For this review, take the finished solid that the model builds, in its own axes (mm). A direction names the side the tool comes from. Give positions to 0.01 mm unless a question says otherwise; leave off trailing zeros. Loops run counter-clockwise (first coordinate to the right, second up) from the corner with the lowest first, then second, coordinate; pieces in that order, holes last. Notation, with made-up numbers: (42.5, -7) - (80.5, -7) arc R23 cw to (80.5, 6) - close; hole circle Ø4 at (33.5, 14). An arc over 180 degrees is marked (long way). Put each result on its own line as item: value. Start each with the question number.
from build123d import *

# Parameters (mm, degrees)
CYLINDER_R              = 3.8
CYLINDER_DEPTH          = 50
CYLINDER001_R           = 10
CYLINDER001_DEPTH       = 15
BOX001_W                = 12
BOX001_H                = 12
BOX001_DEPTH            = 10
BODY003_PLACEMENT_ANGLE = 180
CYLINDER012_R           = 2
CYLINDER012_DEPTH       = 20
ARRAY008_X_COUNT        = 5
ARRAY008_X_PITCH        = 10
CYLINDER013_R           = 1.4
CYLINDER013_DEPTH       = 20
ARRAY009_X_COUNT        = 2
ARRAY009_X_PITCH        = 58
ARRAY010_X_COUNT        = 2
ARRAY010_X_PITCH        = 25
ARRAY010_Y_COUNT        = 2
ARRAY010_Y_PITCH        = 19
BOX011_W                = 30
BOX011_H                = 14
BOX011_DEPTH            = 20
CYLINDER011_R           = 1.8
CYLINDER011_DEPTH       = 20
ARRAY007_X_COUNT        = 2
ARRAY007_X_PITCH        = 68
ARRAY007_Y_COUNT        = 2
ARRAY007_Y_PITCH        = 58
BOX009_W                = 74
BOX009_H                = 64
BOX009_DEPTH            = 3


with BuildPart() as encoder_hole:
    # Cylinder → Cylinder (new body)
    with BuildSketch(Plane.XY):
        Circle(CYLINDER_R)
    extrude(amount=CYLINDER_DEPTH)


with BuildPart() as encoder_cap:
    # Cylinder001 → Cylinder001 (new body)
    with BuildSketch(Plane.XY.offset(35)):
        Circle(CYLINDER001_R)
    extrude(amount=CYLINDER001_DEPTH)


with BuildPart() as encoder_fusion:
    # Box001 → Box001 (new body)
    with BuildSketch(Plane(origin=(-6, -6, 0), x_dir=(1, 0, 0), z_dir=(0, 0, 1))):
        with Locations((6, 6)):
            Rectangle(BOX001_W, BOX001_H)
    extrude(amount=BOX001_DEPTH)

    # Fusion: union encoder hole, encoder cap
    add(encoder_hole.part)
    add(encoder_cap.part)


with BuildPart() as encoder_fusion_1:
    # Fusion placement: moved
    add(encoder_fusion.part.moved(Location((0, 0, -20))))


with BuildPart() as encoder_clone001:
    # Body001 base: copy of encoder fusion
    add(encoder_fusion_1.part)


with BuildPart() as encoder_clone001_1:
    # Clone001 placement: moved
    add(encoder_clone001.part.moved(Location((0, 0, 20))))


with BuildPart() as encoder_clone001_2:
    # Body001 placement: moved
    add(encoder_clone001_1.part.moved(Location((22, 0, -20))))


with BuildPart() as encoder_compound_clone001:
    # Body base: copy of encoder fusion
    add(encoder_fusion_1.part)


with BuildPart() as encoder_compound_clone001_1:
    # Clone placement: moved
    add(encoder_compound_clone001.part.moved(Location((0, 0, 20))))


with BuildPart() as encoder_compound_clone001_2:
    # Body placement: moved
    add(encoder_compound_clone001_1.part.moved(Location((44, 0, -20))))

    # Compound: union encoder clone001, encoder fusion
    add(encoder_clone001_2.part)
    add(encoder_fusion_1.part)


with BuildPart() as encoder_compound_clone001_3:
    # Body003 placement: moved
    add(encoder_compound_clone001_2.part.moved(Location((59, 17, -2))).rotate(Axis((59, 17, -2), (0, 1, 0)), BODY003_PLACEMENT_ANGLE))


with BuildPart() as button_hole_array:
    # Cylinder012 → Cylinder012 (new body)
    with BuildSketch(Plane.XY):
        Circle(CYLINDER012_R)
    extrude(amount=CYLINDER012_DEPTH)

    # Array008 X: button hole array ×5


with BuildPart() as button_hole_array_1:
    add(button_hole_array.part)
    with Locations(*[(i * ARRAY008_X_PITCH, 0, 0) for i in range(1, ARRAY008_X_COUNT)]):
        add(button_hole_array.part)


with BuildPart() as button_hole_array_2:
    # Array008 placement: moved
    add(button_hole_array_1.part.moved(Location((17, 54, -9))))


with BuildPart() as m2_5_bolt_hole:
    # Cylinder013 → Cylinder013 (new body)
    with BuildSketch(Plane.XY):
        Circle(CYLINDER013_R)
    extrude(amount=CYLINDER013_DEPTH)


with BuildPart() as m2_5_bolt_hole_array:
    # Array009 base: copy of m2.5 bolt hole
    add(m2_5_bolt_hole.part)

    # Array009 X: m2.5 bolt hole array ×2


with BuildPart() as m2_5_bolt_hole_array_1:
    add(m2_5_bolt_hole_array.part)
    with Locations(*[(i * ARRAY009_X_PITCH, 0, 0) for i in range(1, ARRAY009_X_COUNT)]):
        add(m2_5_bolt_hole_array.part)


with BuildPart() as m2_5_bolt_hole_array_2:
    # Array009 placement: moved
    add(m2_5_bolt_hole_array_1.part.moved(Location((8, 50, -8))))


with BuildPart() as m2_5_bolt_hole_array001:
    # Body004 base: copy of m2.5 bolt hole
    add(m2_5_bolt_hole.part)

    # Array010 X: m2.5 bolt hole array001 ×2


with BuildPart() as m2_5_bolt_hole_array001_1:
    add(m2_5_bolt_hole_array001.part)
    with Locations(*[(i * ARRAY010_X_PITCH, 0, 0) for i in range(1, ARRAY010_X_COUNT)]):
        add(m2_5_bolt_hole_array001.part)

    # Array010 Y: m2.5 bolt hole array001 ×2


with BuildPart() as m2_5_bolt_hole_array001_2:
    add(m2_5_bolt_hole_array001_1.part)
    with Locations(*[(0, i * ARRAY010_Y_PITCH, 0) for i in range(1, ARRAY010_Y_COUNT)]):
        add(m2_5_bolt_hole_array001_1.part)


with BuildPart() as tft_hole_fusion:
    # Box011 → Box011 (new body)
    with BuildSketch(Plane(origin=(-2.5, 2.5, 0), x_dir=(1, 0, 0), z_dir=(0, 0, 1))):
        with Locations((15, 7)):
            Rectangle(BOX011_W, BOX011_H)
    extrude(amount=BOX011_DEPTH)

    # Fusion006: union m2.5 bolt hole array001
    add(m2_5_bolt_hole_array001_2.part)


with BuildPart() as tft_hole_fusion_1:
    # Fusion006 placement: moved
    add(tft_hole_fusion.part.moved(Location((24.5, 27, -5))))


with BuildPart() as bottom_plate_hole_fusion001:
    # Cylinder011 → Cylinder011 (new body)
    with BuildSketch(Plane(origin=(3, 3, 0), x_dir=(1, 0, 0), z_dir=(0, 0, 1))):
        Circle(CYLINDER011_R)
    extrude(amount=CYLINDER011_DEPTH)

    # Array007 X: bottom plate hole fusion001 ×2


with BuildPart() as bottom_plate_hole_fusion001_1:
    add(bottom_plate_hole_fusion001.part)
    with Locations(*[(i * ARRAY007_X_PITCH, 0, 0) for i in range(1, ARRAY007_X_COUNT)]):
        add(bottom_plate_hole_fusion001.part)

    # Array007 Y: bottom plate hole fusion001 ×2


with BuildPart() as bottom_plate_hole_fusion001_2:
    add(bottom_plate_hole_fusion001_1.part)
    with Locations(*[(0, i * ARRAY007_Y_PITCH, 0) for i in range(1, ARRAY007_Y_COUNT)]):
        add(bottom_plate_hole_fusion001_1.part)

    # Fusion005: union encoder compound clone001, button hole array, m2.5 bolt hole array, tft hole fusion
    add(encoder_compound_clone001_3.part)
    add(button_hole_array_2.part)
    add(m2_5_bolt_hole_array_2.part)
    add(tft_hole_fusion_1.part)


with BuildPart() as top_plate_cut:
    # Box009 → Box009 (new body)
    with BuildSketch(Plane.XY):
        with Locations((37, 32)):
            Rectangle(BOX009_W, BOX009_H)
    extrude(amount=BOX009_DEPTH)

    # Cut006: cut bottom plate hole fusion001
    add(bottom_plate_hole_fusion001_2.part, mode=Mode.SUBTRACT)


solid = top_plate_cut.part
1) Machinability: for faces 1 (the flat face through (37, 43.5, 1)), 2 (the flat face through (0, 32, 1)), which of the approach directions +Z, -Z, +X, -X, +Y, -Y give a long, thin tool a straight path to every point of the face, cutting with its end or side? Answer none if there is none.
2) Wall thickness on probe 1 along Y at (x, z) = (3, 1.85); probe 2 along X at (y, z) = (17, 1.1); probe 3 along X at (y, z) = (46, 0.3): over which ranges is each line inside the solid? List them lowest first.
3) Mouldability with a two-part tool opening along X and no side actions: class faces 3 (the cylindrical face through (24.32, 47.39, 1.48)), 4 (the flat face through (36, 25, 3)), 5 (the flat face through (74, 32, 1)) as released by +X, released by -X, zero draft, split by the parting line, or undercut.
4) Take a section at C-C on z = 0.6. State how many separate pieces and enclosed holes the cut face has, and give its area (3 significant figures).
5) Take a section at A-A on x = 3. State the section outline as (y, z) points.
6) Take a section at B-B on y = 50. State the section outline as (x, z) points.
7) Take a section at D-D on x = 32. State the section outline as (y, z) points.
8) Insertion check: P1, Ø5, axis at x = 37, y = 54, coming from the -Z side. The pin has a flat end and moves straight along its axis. Give the tip position at first contact, or say it passes through.
Answers follow:
1. face 1: +Z, -Z
1. face 2: +Z, -Z, -X, +Y, -Y
2. probe 1: 0 to 1.2, 4.8 to 59.2, 62.8 to 64
2. probe 2: 0 to 11.2, 18.8 to 33.2, 40.8 to 55.2, 62.8 to 74
2. probe 3: 0 to 23.1, 25.9 to 48.1, 50.9 to 74
3. face 3: undercut
3. face 4: zero draft
3. face 5: released by +X
4. separate pieces: 1
4. enclosed holes: 19
4. area: 4,040 mm2
5. outline: (0, 0) - (1.2, 0) - (1.2, 3) - (0, 3) - close; (4.8, 0) - (59.2, 0) - (59.2, 3) - (4.8, 3) - close; (62.8, 0) - (64, 0) - (64, 3) - (62.8, 3) - close
6. outline: (0, 0) - (6.6, 0) - (6.6, 3) - (0, 3) - close; (9.4, 0) - (64.6, 0) - (64.6, 3) - (9.4, 3) - close; (67.4, 0) - (74, 0) - (74, 3) - (67.4, 3) - close
7. outline: (0, 0) - (29.5, 0) - (29.5, 3) - (0, 3) - close; (43.5, 0) - (64, 0) - (64, 3) - (43.5, 3) - close
8. P1: z = 0
